```python
from build123d import *

# Parameters (mm, degrees)
SKETCH1_W           = 8
SKETCH1_H           = 16
BOSS_EXTRUDE1_DEPTH = 3
SKETCH3_R           = 2.5
CUT_EXTRUDE1_DEPTH  = 10
SKETCH2_W           = 3
SKETCH2_H           = 3
BOSS_EXTRUDE3_DEPTH = 4


with BuildPart() as part:
    # Sketch1 → Boss-Extrude1 (new body)
    with BuildSketch(Plane.XY):
        with Locations((4, 8)):
            Rectangle(SKETCH1_W, SKETCH1_H)
    extrude(amount=BOSS_EXTRUDE1_DEPTH)

    # Sketch3 → Cut-Extrude1 (cut)
    with BuildSketch(Plane.XY.offset(3)):
        with Locations((3.98651131, 12.5)):
            Circle(SKETCH3_R)
    extrude(amount=-CUT_EXTRUDE1_DEPTH, mode=Mode.SUBTRACT)

    # Sketch2 → Boss-Extrude3 (add)
    with BuildSketch(Plane.ZY):
        with Locations((1.5, 2.5)):
            Rectangle(SKETCH2_W, SKETCH2_H)
    extrude(amount=BOSS_EXTRUDE3_DEPTH)


solid = part.part
```
Can you work these out from the model? Positions are in its coordinate system, mm. A direction names the side the tool comes from. Round coordinates to 2 decimals unless told otherwise and drop trailing zeros. Loops run counter-clockwise (first coordinate to the right, second up) from the corner with the lowest first, then second, coordinate; pieces in that order, holes last.
Item 1: Please list where these lines run through material, in increasing order: L1, parallel to Y at x = -2, z = 0.6; L2, parallel to Y at x = 5.75, z = 1; L3, parallel to X at y = 4.5, z = 1.9.
Item 2: Suppose I cut it at A-A, the plane z = 1.25. Write out the boundary of the cut face in (x, y), then the cut area to 3 significant figures.
Item 3: Suppose I cut it at C-C, the plane x = 4.5. Write out the boundary of the cut face in (y, z).
Item 4: Will this pin go through, and if not, where does the flat tip stop? pin 1 Ø3 at (x, y) = (3.99, 12.5) entering from +Z (1 decimal).
Item 5: Suppose I cut it at D-D, the plane y = 9. Write out the boundary of the cut face in (x, z).
Item 6: Which directions (+Z, -Z, +X, -X, +Y, -Y) give clear straight access to the entire face, cutting with the end or side of a thin tool? Please do faces 1 (the flat face through (4, 0, 1)), 2 (the flat face through (0, 0.5, 1.5)), 3 (the flat face through (0, 10, 1)).
Item 7: Suppose I cut it at B-B, the plane y = 12.5. Write out the boundary of the cut face in (x, z).
Item 8: If we mould it in two halves opening along X, with no side actions, what happens to faces 4 (the cylindrical face through (3.44, 10.06, 1.52)), 5 (the flat face through (8, 8, 1)), 6 (the flat face through (-2, 4, 1))? For each: +X half, -X half, draft (parallel to the pull), parting line (faces both ways), or undercut.
Reported:
1. L1: y = 1 to 4
1. L2: y = 0 to 10.73, 14.27 to 16
1. L3: x = 0 to 8
2. outline: (-4, 1) - (0, 1) - (0, 0) - (8, 0) - (8, 16) - (0, 16) - (0, 4) - (-4, 4) - close; hole circle Ø5 at (3.99, 12.5)
2. area: 120 mm2
3. outline: (0, 0) - (10.05, 0) - (10.05, 3) - (0, 3) - close; (14.95, 0) - (16, 0) - (16, 3) - (14.95, 3) - close
4. pin 1: passes through
5. outline: (0, 0) - (8, 0) - (8, 3) - (0, 3) - close
6. face 1: +Z, -Z, +X, -X, -Y
6. face 2: +Z, -Z, -X, -Y
6. face 3: +Z, -Z, -X, +Y
7. outline: (0, 0) - (1.49, 0) - (1.49, 3) - (0, 3) - close; (6.49, 0) - (8, 0) - (8, 3) - (6.49, 3) - close
8. face 4: undercut
8. face 5: +X half
8. face 6: draft
